from build123d import *

# Parameters (mm, degrees)
EXTRUDE_1_DEPTH = 2


with BuildPart() as part:
    # Эскиз1 → Бобышка-Вытянуть1 (new body)
    with BuildSketch(Plane(origin=(0, 0, 0), x_dir=(1, 0, 0), z_dir=(0, 1, 0))):
        with BuildLine():
            Line((40.5, -11.5), (-40.5, -11.5))
            ThreePointArc((-40.5, -11.5), (-41.914213562, -10.914213562), (-42.5, -9.5))
            Line((-42.5, -9.5), (-42.5, 9.5))
            ThreePointArc((-42.5, 9.5), (-41.914213562, 10.914213562), (-40.5, 11.5))
            Line((-40.5, 11.5), (40.5, 11.5))
            ThreePointArc((40.5, 11.5), (41.914213562, 10.914213562), (42.5, 9.5))
            Line((42.5, 9.5), (42.5, -9.5))
            ThreePointArc((42.5, -9.5), (41.914213562, -10.914213562), (40.5, -11.5))
        make_face()
        with BuildLine():
            ThreePointArc((-30, 6), (-36, 0), (-30, -6))
            ThreePointArc((-30, -6), (-24, 0), (-30, 6))
        make_face(mode=Mode.SUBTRACT)
        with BuildLine():
            ThreePointArc((30, 6), (36, 0), (30, -6))
            ThreePointArc((30, -6), (24, 0), (30, 6))
        make_face(mode=Mode.SUBTRACT)
    extrude(amount=EXTRUDE_1_DEPTH)


solid = part.part
Could you check a few things on this model? Use its own coordinates, in mm. Give positions to 0.01 mm unless a question says otherwise; leave off trailing zeros. Loops run counter-clockwise (first coordinate to the right, second up) from the corner with the lowest first, then second, coordinate; pieces in that order, holes last. Notation, with made-up numbers: M 61,34 L 79,34 A19 ccw 79,48 Z; hole C 62.5,6.5 d4. An arc over 180 degrees is marked long. Answer as a JSON object with one key per item and string values.
Q1. For P1, Ø2, axis at x = -8.5, z = 1.5, coming from the -Y side, with a flat end and sliding along its axis, tell me the tip position at first contact or that it passes through.
Values found:
{"P1": "stops at y = 0"}
Q2. If we mould it in two halves opening along Z, with no side actions, what happens to faces 1 (the cylindrical face through (-41.9, 0.99, 10.93)), 2 (the flat face through (42.5, 1, 0)), 3 (the cylindrical face through (35.857, 0.986, -1.301)), 4 (the cylindrical face through (-35.857, 0.986, -1.301))? For each: pulls with the +Z half, pulls with the -Z half, needs draft (parallel to the pull), parting line crosses it, or undercut.
Values found:
{"face 1": "pulls with the +Z half", "face 2": "needs draft", "face 3": "undercut", "face 4": "undercut"}
Q3. Suppose I cut it at D-D, the plane z = 4. List the corners of the cut face in (x, y) for me, plus the area to 3 significant figures.
Values found:
{"outline": "M -42.5,0 L -34.47,0 L -34.47,2 L -42.5,2 Z; M -25.53,0 L 25.53,0 L 25.53,2 L -25.53,2 Z; M 34.47,0 L 42.5,0 L 42.5,2 L 34.47,2 Z", "area": "134 mm²"}
Q4. Suppose I cut it at A-A, the plane x = -30. List the corners of the cut face in (y, z) for me, plus the area to 3 significant figures.
Values found:
{"outline": "M 0,-11.5 L 2,-11.5 L 2,-6 L 0,-6 Z; M 0,6 L 2,6 L 2,11.5 L 0,11.5 Z", "area": "22.0 mm²"}
Q5. If I drill on probe 1 along X at (y, z) = (1.4, 0); probe 2 along Z at (x, y) = (30, 0.55); probe 3 along X at (y, z) = (0.6, -5), over which ranges is the centre line in solid material (lowest first)? Write a range as [from, to].
Values found:
{"probe 1": "x = [-42.5, -36], [-24, 24], [36, 42.5]", "probe 2": "z = [-11.5, -6], [6, 11.5]", "probe 3": "x = [-42.5, -33.32], [-26.68, 26.68], [33.32, 42.5]"}
Q6. Suppose I cut it at C-C, the plane z = -2.75. List the corners of the cut face in (x, y) for me.
Values found:
{"outline": "M -42.5,0 L -35.33,0 L -35.33,2 L -42.5,2 Z; M -24.67,0 L 24.67,0 L 24.67,2 L -24.67,2 Z; M 35.33,0 L 42.5,0 L 42.5,2 L 35.33,2 Z"}
Q7. Suppose I cut it at B-B, the plane y = 0.5. List the corners of the cut face in (x, z) for me, plus the area to 3 significant figures.
Values found:
{"outline": "M -42.5,-9.5 A2 ccw -40.5,-11.5 L 40.5,-11.5 A2 ccw 42.5,-9.5 L 42.5,9.5 A2 ccw 40.5,11.5 L -40.5,11.5 A2 ccw -42.5,9.5 Z; hole C -30,0 d12; hole C 30,0 d12", "area": "1,730 mm²"}
